Geometry: final body of the model. Coordinates: model frame, mm. Face numbers are marked on the shaded views. A direction names the side the tool comes from. Round coordinates to 2 decimals unless told otherwise and drop trailing zeros. Loops run counter-clockwise (first coordinate to the right, second up) from the corner with the lowest first, then second, coordinate; pieces in that order, holes last. Notation, with made-up numbers: M 74.25,72.5 L 103.25,72.5 A16 ccw 103.25,77.5 Z; hole C 12.5,17.5 d11. An arc over 180 degrees is marked long. Answer as a JSON object with one key per item and string values.
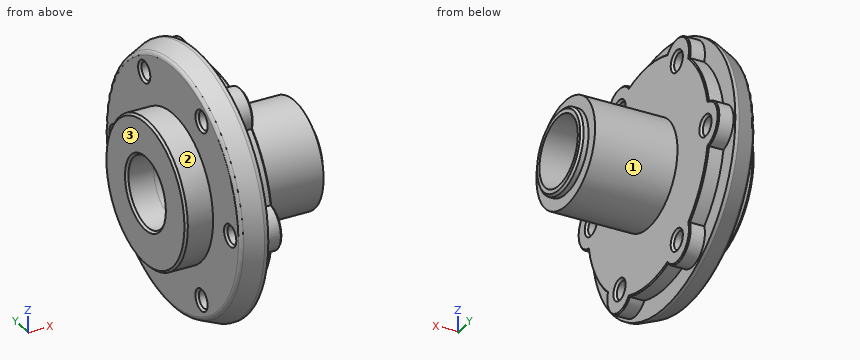
from build123d import *
from build123d.topology import SkipClean

# Parameters (mm, degrees)
SKETCH2_R                    = 12.7635
BOSS_EXTRUDE1_DEPTH          = 19.05
SKETCH3_R                    = 9.4615
BOSS_EXTRUDE2_DEPTH          = 1.651
F_5_8_0_628_DIAMETER_HOLE1_D = 15.9512
F_21_0_159_DIAMETER_HOLE1_D  = 4.0386
F_21_0_159_DIAMETER_HOLE2_D  = 4.0386
CHAMFER1_SIZE                = 0.508000007
FILLET1_R                    = 1.016
FILLET2_R                    = 2.54
SKETCH10_R                   = 29.845
CUT_EXTRUDE1_DEPTH           = 3.556
CHAMFER3_SIZE                = 0.254
SKETCH12_R                   = 33.252215347
SKETCH12_R_2                 = 12.192
OUTSIDE_BORE_TRIM_DEPTH      = 20.701
SKETCH15_R                   = 16.7132
SKETCH15_R_2                 = 7.9756
BOSS_EXTRUDE5_DEPTH          = 6.35
CHAMFER6_SIZE                = 0.508


with BuildPart() as part:
    # Sketch1 → Revolve1 (revolve)
    with BuildSketch(Plane(origin=(0, 0, 0), x_dir=(-1, 0, 0), z_dir=(0, 0, -1)), mode=Mode.PRIVATE) as revolve1_sk:
        Polygon((-55.88, 29.845), (-55.88, 0), (-46.863, 0), (-46.863, 27.94), (-51.462076836, 29.845), align=None)
    revolve(revolve1_sk.sketch.rotate(Axis((55.88, 0, 0), (-1, 0, 0)), 270), axis=Axis((55.88, 0, 0), (-1, 0, 0)))

    # Sketch2 → Boss-Extrude1 (add)
    with BuildSketch(Plane(origin=(55.88, 0, 0), x_dir=(0, 0, -1), z_dir=(1, 0, 0))):
        with Locations(Location((0, 0, 0), (0, 0, 180))):
            Circle(SKETCH2_R)
    extrude(amount=BOSS_EXTRUDE1_DEPTH)

    # Sketch3 → Boss-Extrude2 (add)
    with BuildSketch(Plane(origin=(74.93, 0, 0), x_dir=(0, 0, -1), z_dir=(1, 0, 0))):
        Circle(SKETCH3_R)
    extrude(amount=BOSS_EXTRUDE2_DEPTH)

    # 5/8 (0.628) Diameter Hole1 (through all)
    with Locations(Plane.ZY.offset(-46.863)):
        with Locations((0, 0)):
            Hole(F_5_8_0_628_DIAMETER_HOLE1_D / 2)

    # #21 (0.159) Diameter Hole1 (through all)
    with Locations(Plane(origin=(55.88, 0, 0), x_dir=(0, 0, -1), z_dir=(1, 0, 0))):
        with Locations((-20.622229928, 11.90625), (20.622229928, 11.90625), (20.622229928, -11.90625), (0, -23.8125)):
            Hole(F_21_0_159_DIAMETER_HOLE1_D / 2)

    # #21 (0.159) Diameter Hole2 (through all)
    with Locations(Plane.ZY.offset(-46.863)):
        with Locations((20.622229928, -11.90625), (0, 23.8125)):
            Hole(F_21_0_159_DIAMETER_HOLE2_D / 2)

    # Chamfer1
    chamfer1_edges = [part.edges().sort_by_distance(p)[0] for p in [
        (74.93, 0, -12.7635),
        (76.581, 0, 9.4615),
        (55.88, -23.8125, -2.0193),
        (46.863, -23.8125, -2.0193),
        (55.88, -11.90625, -22.641529928),
        (46.863, -11.90625, -22.641529928),
        (55.88, 11.90625, -22.641529928),
        (46.863, 11.90625, -22.641529928),
        (55.88, 11.90625, 18.602929928),
        (46.863, 11.90625, 18.602929928),
        (55.88, 23.8125, 2.0193),
        (46.863, 23.8125, 2.0193),
        (55.88, -11.90625, 22.641529928),
        (46.863, -11.90625, 22.641529928),
    ]]
    chamfer(chamfer1_edges, length=CHAMFER1_SIZE)

    # Fillet1
    fillet1_edges = [part.edges().sort_by_distance(p)[0] for p in [
        (46.863, 0, -27.94),
    ]]
    fillet(fillet1_edges, radius=FILLET1_R)

    # Fillet2
    fillet2_edges = [part.edges().sort_by_distance(p)[0] for p in [
        (55.88, 0, -12.7635),
    ]]
    fillet(fillet2_edges, radius=FILLET2_R)

    # Sketch10 → Cut-Extrude1 (cut)
    with BuildSketch(Plane(origin=(55.88, 0, 0), x_dir=(0, 0, -1), z_dir=(1, 0, 0))):
        with Locations(Location((0, 0, 0), (0, 0, 180))):
            Circle(SKETCH10_R)
        with BuildLine():
            ThreePointArc((5.194684655, 24.894464178), (12.71872072, 22.021653827), (18.96710386, 16.940131795))
            ThreePointArc((18.96710386, 16.940131795), (25.217002518, 14.554101773), (24.156474078, 7.94882722))
            ThreePointArc((24.156474078, 7.94882722), (25.430672133, -0.003203872), (24.154470478, -7.954913657))
            ThreePointArc((24.154470478, -7.954913657), (25.213334557, -14.560455175), (18.962834963, -16.944910398))
            ThreePointArc((18.962834963, -16.944910398), (12.713171601, -22.024857913), (5.188411857, -24.895772345))
            ThreePointArc((5.188411857, -24.895772345), (-0.002445392, -29.114749939), (-5.19259389, -24.894900477))
            ThreePointArc((-5.19259389, -24.894900477), (-12.717500776, -22.022358557), (-18.966649715, -16.940640514))
            ThreePointArc((-18.966649715, -16.940640514), (-25.214891362, -14.55429486), (-24.156019778, -7.950208229))
            ThreePointArc((-24.156019778, -7.950208229), (-25.430672245, 0.003203856), (-24.154015788, 7.956294514))
            ThreePointArc((-24.154015788, 7.956294514), (-25.21122333, 14.560647771), (-18.962380547, 16.945418955))
            ThreePointArc((-18.962380547, 16.945418955), (-12.711951385, 22.02556217), (-5.186321013, 24.896207969))
            ThreePointArc((-5.186321013, 24.896207969), (0.004890594, 29.114749631), (5.194684655, 24.894464178))
        make_face(mode=Mode.SUBTRACT)
    extrude(amount=-CUT_EXTRUDE1_DEPTH, mode=Mode.SUBTRACT)

    # Chamfer3
    chamfer3_edges = [part.edges().sort_by_distance(p)[0] for p in [
        (55.88, 14.554101773, -25.217002518),
        (55.88, 22.021653827, -12.71872072),
        (55.88, 29.114749631, -0.004890594),
        (55.88, 22.02556217, 12.711951385),
        (55.88, 14.560647771, 25.21122333),
        (55.88, 0.003203856, 25.430672245),
        (55.88, -14.55429486, 25.214891362),
        (55.88, -22.022358557, 12.717500776),
        (55.88, -29.114749939, 0.002445392),
        (55.88, -22.024857913, -12.713171601),
        (55.88, -14.560455175, -25.213334557),
        (55.88, -0.003203872, -25.430672133),
    ]]
    chamfer(chamfer3_edges, length=CHAMFER3_SIZE)

    # Sketch12 → Outside Bore Trim (cut)
    with BuildSketch(Plane(origin=(76.581, 0, 0), x_dir=(0, 0, -1), z_dir=(1, 0, 0))):
        Circle(SKETCH12_R)
        Circle(SKETCH12_R_2, mode=Mode.SUBTRACT)
    extrude(amount=-OUTSIDE_BORE_TRIM_DEPTH, mode=Mode.SUBTRACT)

    # Sketch15 → Boss-Extrude5 (add)
    with SkipClean():  # the faces are left unmerged after this step: merging them gives an invalid solid
        with BuildSketch(Plane.ZY.offset(-46.863)):
            Circle(SKETCH15_R)
            Circle(SKETCH15_R_2, mode=Mode.SUBTRACT)
        extrude(amount=BOSS_EXTRUDE5_DEPTH)
    add(part.part.scale(1), mode=Mode.REPLACE)  # the faces are merged on a copy

    # Chamfer6
    chamfer6_edges = [part.edges().sort_by_distance(p)[0] for p in [
        (40.513, 0, -16.7132),
        (40.513, 0, -7.9756),
    ]]
    chamfer(chamfer6_edges, length=CHAMFER6_SIZE)


solid = part.part
1) Ray query, line 1 (Y direction, x = 53, z = 0); line 2 (Y direction, x = 51, z = 0); line 3 (Y direction, x = 44.25, z = 0). Return the intervals inside material, ascending.
Results:
{"line 1": "-29.11 to -25.83, -21.79 to -7.98, 7.98 to 21.79, 25.83 to 29.11", "line 2": "-29.65 to -25.83, -21.79 to -7.98, 7.98 to 21.79, 25.83 to 29.65", "line 3": "-16.71 to -7.98, 7.98 to 16.71"}
2) Reachability of the marked faces 1, 2 and 3 from +Z, -Z, +X, -X, +Y, -Y: full face, straight path, thin tool, end or side. Return the list, or none.
Results:
{"face 1": "+X", "face 2": "-X", "face 3": "+Z, -Z, -X, +Y, -Y"}
3) Pin query (flat end, axial travel): P1, Ø15.5, axis at y = 4.5, z = -0.5, coming from the +X side; P2, Ø6.5, axis at y = 11.91, z = -20.62, coming from the +X side; P3, Ø12, axis at x = 61, z = 4, coming from the +Y side; P4, Ø1.5, axis at x = 65.5, z = -11.5, coming from the +Y side. Return the tip coordinate at first contact, or that it passes through.
Results:
{"P1": "x = 76.58", "P2": "x = 55.88", "P3": "y = 28.94", "P4": "y = 5.75"}
4) Section query B-B (z = 0). Count the separate pieces of the cut face and the enclosed holes in it, and give its area (3 significant figures).
Results:
{"separate pieces": "4", "enclosed holes": "0", "area": "582 mm2"}
5) Section query A-A (x = 44). Return the cut outline in (y, z).
Results:
{"outline": "C 0,0 d33.43; hole C 0,0 d15.95"}
6) Section query D-D (x = 50). Return the cut outline in (y, z), and give its area (3 significant figures).
Results:
{"outline": "C 0,0 d58.48; hole C -23.81,0 d4.04; hole C -11.91,-20.62 d4.04; hole C -11.91,20.62 d4.04; hole C 0,0 d15.95; hole C 11.91,-20.62 d4.04; hole C 11.91,20.62 d4.04; hole C 23.81,0 d4.04", "area": "2,410 mm2"}
